```python
from build123d import *

# Parameters (mm, degrees)
F0_W     = 4
F0_H     = 8
F3_START = -55
F2_W     = 10.6760558783
F2_H     = 2
F2_W_2   = 2
F2_H_2   = 10.1549292555
F3_DEPTH = 18


with BuildPart() as f1:
    # F0 (on Top) → F1 (revolve)
    with BuildSketch(Plane.XY):
        Polygon((0, 73), (0, 68), (4, 68), (5, 68), (3, 73), align=None)
        with Locations((2, 64)):
            Rectangle(F0_W, F0_H)
        Polygon((0, 60), (0, 0), (5, 0), (5, 60), (4, 60), align=None)
    revolve(axis=Axis((0, 30, 0), (0, -1, 0)))

    # F2 (on Front) → F3 (cut)
    with BuildSketch(Plane.XZ.offset(F3_START)):
        with Locations((-6.3380279391, 0)):
            Rectangle(F2_W, F2_H)
        Rectangle(F2_W_2, F2_H)
        with Locations((0, 6.0774646278)):
            Rectangle(F2_W_2, F2_H_2)
        with Locations((6.3380279391, 0)):
            Rectangle(F2_W, F2_H)
        with Locations((0, -6.0774646278)):
            Rectangle(F2_W_2, F2_H_2)
    extrude(amount=-F3_DEPTH, mode=Mode.SUBTRACT)

    # F4: F1 across face


with BuildPart() as f1_1:
    add(f1.part)
    add(f1.part.mirror(Plane.XZ))


solid = f1_1.part
```
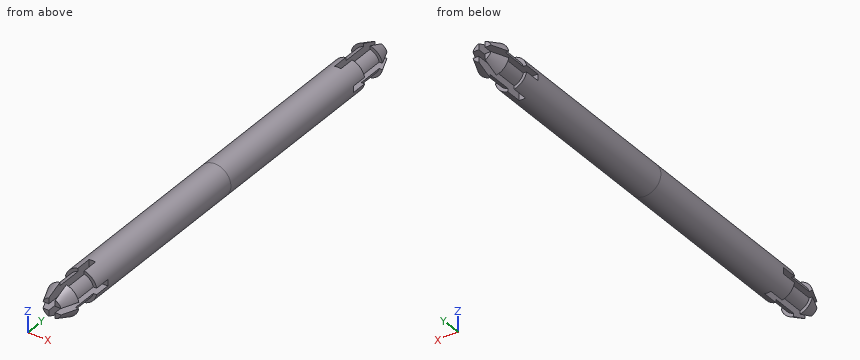
Work out the finished part from the listing and answer in its coordinate system (mm). Round coordinates to 2 decimals unless told otherwise and drop trailing zeros. Write each loop counter-clockwise with the first axis right and the second up, starting at its lowest first coordinate (ties: lowest second). Pieces come first, ordered by that corner, then holes. Notation, with made-up numbers: (79, 87) - (105, 87) arc R24 ccw to (105, 115) - close; hole circle Ø7 at (9.5, 83.5). An arc over 180 degrees is marked (long way). Return JSON: item names as keys, results as strings. Group by question number.
Q1. Find the intervals of material crossed by L1, parallel to Y at x = 4, z = -2.25; L2, parallel to Z at x = -0.25, y = -3.5; L3, parallel to Y at x = 0.25, z = -2, in increasing order.
Q2. Each of these flat-tipped pins is pushed along its axis until it touches: pin 1 Ø1.2 at (x, z) = (-2.5, 3) entering from +Y; pin 2 Ø1.2 at (x, z) = (-3.5, -2.5) entering from -Y; pin 3 Ø1 at (x, y) = (2.5, -28.5) entering from -Z; pin 4 Ø4.5 at (x, z) = (2, 4) entering from -Y. Where does it stop, or does it pass through?
Q3. The part is cut by section A-A on y = -32.5. Write down the section's boundary in (x, z).
Solved:
{
 "1": {"L1": "-69.03 to -68, -60 to 60, 68 to 69.03", "L2": "-4.99 to 4.99", "L3": "-55 to 55"},
 "2": {"pin 1": "y = 72.24", "pin 2": "y = -71.25", "pin 3": "z = -4.58", "pin 4": "y = -73"},
 "3": {"outline": "circle Ø10 at (0, 0)"}
}
